Part model, mm, in its own coordinate system. A direction names the side the tool comes from. Give positions to 0.01 mm unless a question says otherwise; leave off trailing zeros. Loops run counter-clockwise (first coordinate to the right, second up) from the corner with the lowest first, then second, coordinate; pieces in that order, holes last. Notation, with made-up numbers: M 1.25,10 L 5.25,10 A20 ccw 5.25,17 Z; hole C 58,17.25 d6. An arc over 180 degrees is marked long. Put each result on its own line as item: value. Start each with the question number.
```python
from build123d import *

# Parameters (mm, degrees)
F1_DEPTH = 3
F2_R     = 2
F3_DEPTH = 25


with BuildPart() as f1:
    # F0 (on Top) → F1 (new body)
    with BuildSketch(Plane.XY):
        with BuildLine():
            Line((63.5, 3), (-63.5, 3))
            ThreePointArc((-63.5, 3), (-72.5, 0), (-63.5, -3))
            Line((-63.5, -3), (63.5, -3))
            ThreePointArc((63.5, -3), (72.5, 0), (63.5, 3))
        make_face()
    extrude(amount=F1_DEPTH)

    # F2 (on Top) → F3 (cut)
    with BuildSketch(Plane.XY):
        with Locations((67.5, 0)):
            Circle(F2_R)
        with Locations((-67.5, 0)):
            Circle(F2_R)
    extrude(amount=F3_DEPTH, mode=Mode.SUBTRACT)


solid = f1.part
```
1) Band-saw the part on B-B on x = 67.5. Give the cut face in (y, z), then the cut area to 3 significant figures.
2) Mould opens along X. For faces 1 (the flat face through (-1, 0, 3)), 2 (the cylindrical face through (72.497, -0.175, 1.479)) say: +X half, -X half, draft (parallel to the pull), parting line (faces both ways), or undercut.
3) Which spindle directions (+Z, -Z, +X, -X, +Y, -Y) get a long thin tool onto all of the face, cutting with end or side? Do faces 3 (the cylindrical face through (-65.592, 0.601, 1.479)), 4 (the flat face through (-1, -3, 1)), 5 (the flat face through (1, 3, 1)). Say none if no direction does.
4) Band-saw the part on A-A on y = 0. Give the cut face in (x, z).
5) Band-saw the part on C-C on z = 2.45. Give the cut face in (x, y), then the cut area to 3 significant figures.
6) Wall check: L1, parallel to X at y = 0, z = 2.2; L2, parallel to X at y = -0.75, z = 1.8; L3, parallel to Y at x = 67.5, z = 1. Give the ranges that are in metal, low to high.
7) Band-saw the part on D-D on x = -60. Give the cut face in (y, z), then the cut area to 3 significant figures.
8) Pin check, flat tips, straight feed: pin 1 Ø1.5 at (x, z) = (34, 2.5) entering from -Y; pin 2 Ø3 at (x, y) = (-67.5, 0) entering from +Z; pin 3 Ø1 at (x, z) = (18, 2) entering from +Y. Stop position of each tip, or through.
Evaluation:
1. outline: M -5,0 L -2,0 L -2,3 L -5,3 Z; M 2,0 L 5,0 L 5,3 L 2,3 Z
1. area: 18.0 mm2
2. face 1: draft
2. face 2: undercut
3. face 3: +Z, -Z
3. face 4: +Z, -Z, -Y
3. face 5: +Z, -Z, +Y
4. outline: M -72.5,0 L -69.5,0 L -69.5,3 L -72.5,3 Z; M -65.5,0 L 65.5,0 L 65.5,3 L -65.5,3 Z; M 69.5,0 L 72.5,0 L 72.5,3 L 69.5,3 Z
5. outline: M -63.5,-3 L 63.5,-3 A5 ccw long 63.5,3 L -63.5,3 A5 ccw long Z; hole C -67.5,0 d4; hole C 67.5,0 d4
5. area: 886 mm2
6. L1: -72.5 to -69.5, -65.5 to 65.5, 69.5 to 72.5
6. L2: -72.44 to -69.35, -65.65 to 65.65, 69.35 to 72.44
6. L3: -5 to -2, 2 to 5
7. outline: M -3,0 L 3,0 L 3,3 L -3,3 Z
7. area: 18.0 mm2
8. pin 1: y = -3
8. pin 2: through
8. pin 3: y = 3
